Job drawing, mm, ordinate dimensions from the low corner. One solid piece. Coordinates: 2 decimals unless noted, no trailing zeros. Loops run counter-clockwise (first coordinate to the right, second up) from the corner with the lowest first, then second, coordinate; pieces in that order, holes last. Notation, with made-up numbers: (-23, -5) -> (8, -5) arc R20 cw to (8, 13) -> close; hole circle Ø1 at (-15.75, 74). An arc over 180 degrees is marked (long way). Use one line per item in the form item = value. Start each with the question number.
(1) Band-saw the part on A-A on x = 8. Give the cut face in (y, z).
(2) Pin check, flat tips, straight feed: P1, Ø5, axis at x = 4.5, y = 12, coming from the +Z side; P2, Ø6, axis at x = 8, z = 8, coming from the +Y side; P3, Ø1.5, axis at y = 21.5, z = 13.5, coming from the -X side. Stop position of each tip, or through.
(3) Band-saw the part on C-C on y = 14.5. Give the cut face in (x, z), then the cut area to 3 significant figures.
(4) Band-saw the part on B-B on z = 6.5. Give the cut face in (x, y).
(5) Mould opens along X. For the marked faces 1, 2 and 3 say: +X half, -X half, draft (parallel to the pull), parting line (faces both ways), or undercut.
(6) Band-saw the part on D-D on x = 12.75. Give the cut face in (y, z), then the cut area to 3 significant figures.
(7) Drill centre lines: L1, parallel to Z at x = 8, y = 20.25; L2, parallel to X at y = 7.25, z = 7.75; L3, parallel to X at y = 15.25, z = 10.5. Where is each one in solid material? Low to high. Write a range as [from, to].
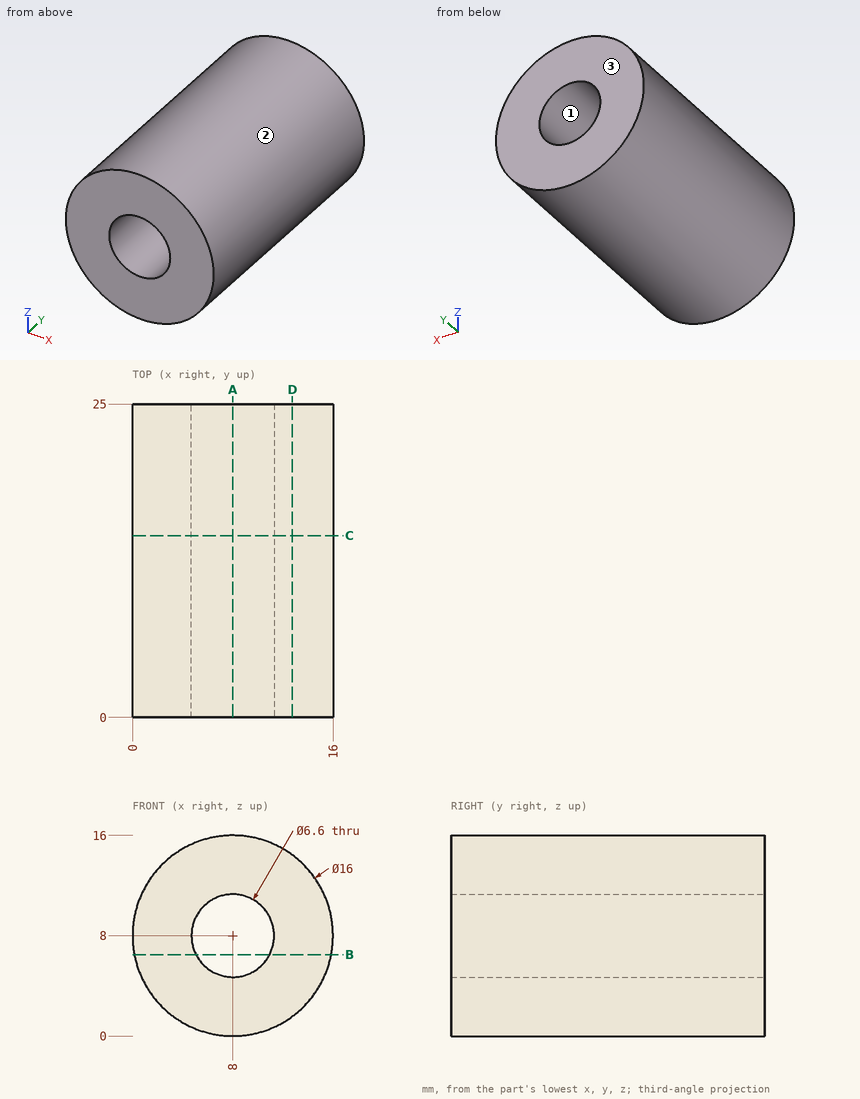
A:
q1.outline = (0, 0) -> (25, 0) -> (25, 4.7) -> (0, 4.7) -> close; (0, 11.3) -> (25, 11.3) -> (25, 16) -> (0, 16) -> close
q2.P1 = 15.94
q2.P2 = through
q2.P3 = 1.56
q3.outline = circle Ø16 at (8, 8); hole circle Ø6.6 at (8, 8)
q3.area = 167 mm²
q4.outline = (0.14, 0) -> (5.06, 0) -> (5.06, 25) -> (0.14, 25) -> close; (10.94, 0) -> (15.86, 0) -> (15.86, 25) -> (10.94, 25) -> close
q5.face_1 = undercut
q5.face_2 = parting line
q5.face_3 = draft
q6.outline = (0, 1.56) -> (25, 1.56) -> (25, 14.44) -> (0, 14.44) -> close
q6.area = 322 mm²
q7.L1 = [0, 4.7], [11.3, 16]
q7.L2 = [0, 4.71], [11.29, 16]
q7.L3 = [0.4, 5.85], [10.15, 15.6]
